from build123d import *

# Parameters (mm, degrees)
SKETCH2_W                       = 125
SKETCH2_H                       = 35
SKETCH2_R                       = 10
BOSS_EXTRUDE1_DEPTH             = 5
BOSS_EXTRUDE3_REACH             = 19.5
BOSS_EXTRUDE3_DIRECTION_2_REACH = 19.5
CUT_EXTRUDE2_DEPTH              = 12.5
CUT_EXTRUDE2_DEPTH_BACK         = 12.5
SKETCH8_R                       = 12.75
SKETCH8_R_2                     = 10.25
BOSS_EXTRUDE4_DEPTH             = 30.2
FILLET1_R                       = 5
SKETCH9_R                       = 3.5
CUT_EXTRUDE3_DEPTH              = 36.0000001
SKETCH13_R                      = 2
CUT_EXTRUDE5_DEPTH              = 2.5
CUT_EXTRUDE6_DEPTH              = 6
BOSS_EXTRUDE7_DEPTH             = 72
SKETCH17_R                      = 7.5
BOSS_EXTRUDE8_DEPTH             = 4
SKETCH18_R                      = 10.25
BOSS_EXTRUDE9_DEPTH             = 9.5


with BuildPart() as part:
    # Sketch2 → Boss-Extrude1 (new body)
    with BuildSketch(Plane(origin=(0, 0, 0), x_dir=(1, 0, 0), z_dir=(0, 1, 0))):
        Rectangle(SKETCH2_W, SKETCH2_H)
        with Locations((-25, 0)):
            Circle(SKETCH2_R, mode=Mode.SUBTRACT)
    extrude(amount=BOSS_EXTRUDE1_DEPTH)

    # Boss-Extrude3: up to this face of the body (flat: up to its plane)
    boss_extrude3_end = Plane(part.part.faces().sort_by_distance((0, 2.5, -17.5))[0])
    # Sketch6 → Boss-Extrude3 (add, up to the picked face)
    with BuildSketch(Plane.XY, mode=Mode.PRIVATE) as boss_extrude3_sk1:
        with BuildLine():
            Line((-62.5, 5), (-4.580943715, 34.11344911))
            ThreePointArc((-4.580943715, 34.11344911), (0, 35.2), (4.580943715, 34.11344911))
            Line((4.580943715, 34.11344911), (62.5, 5))
            Line((62.5, 5), (-62.5, 5))
        make_face()
    boss_extrude3_tool1 = split(extrude(boss_extrude3_sk1.sketch, amount=-BOSS_EXTRUDE3_REACH, mode=Mode.PRIVATE), bisect_by=boss_extrude3_end, keep=Keep.BOTH, mode=Mode.PRIVATE)
    add(boss_extrude3_tool1.solids().sort_by_distance((0, 15.43289, 0))[0])

    # Boss-Extrude3 direction 2: up to this face of the body (flat: up to its plane)
    boss_extrude3_direction_2_end = Plane(part.part.faces().sort_by_distance((0, 2.5, 17.5))[0])
    # Sketch6 → Boss-Extrude3 direction 2 (add, up to the picked face)
    with BuildSketch(Plane.XY, mode=Mode.PRIVATE) as boss_extrude3_direction_2_sk1:
        with BuildLine():
            Line((-62.5, 5), (-4.580943715, 34.11344911))
            ThreePointArc((-4.580943715, 34.11344911), (0, 35.2), (4.580943715, 34.11344911))
            Line((4.580943715, 34.11344911), (62.5, 5))
            Line((62.5, 5), (-62.5, 5))
        make_face()
    boss_extrude3_direction_2_tool1 = split(extrude(boss_extrude3_direction_2_sk1.sketch, amount=BOSS_EXTRUDE3_DIRECTION_2_REACH, mode=Mode.PRIVATE), bisect_by=boss_extrude3_direction_2_end, keep=Keep.BOTH, mode=Mode.PRIVATE)
    add(boss_extrude3_direction_2_tool1.solids().sort_by_distance((0, 15.43289, 0))[0])

    # Sketch7 → Cut-Extrude2 (cut, two sides)
    with BuildSketch(Plane.XY) as cut_extrude2_sk:
        with BuildLine():
            Line((4.580943715, 34.11344911), (62.5, 5))
            Line((62.5, 5), (-62.5, 5))
            Line((-62.5, 5), (-4.580943715, 34.11344911))
            ThreePointArc((-4.580943715, 34.11344911), (0, 35.2), (4.580943715, 34.11344911))
        make_face()
    extrude(amount=CUT_EXTRUDE2_DEPTH, mode=Mode.SUBTRACT)
    extrude(cut_extrude2_sk.sketch, amount=-CUT_EXTRUDE2_DEPTH_BACK, mode=Mode.SUBTRACT)

    # Sketch8 → Boss-Extrude4 (add)
    with BuildSketch(Plane(origin=(0, 5, 0), x_dir=(1, 0, 0), z_dir=(0, 1, 0))):
        Circle(SKETCH8_R)
        Circle(SKETCH8_R_2, mode=Mode.SUBTRACT)
    extrude(amount=BOSS_EXTRUDE4_DEPTH)

    # Fillet1
    fillet1_edges = [part.edges().sort_by_distance(p)[0] for p in [
        (0, 0, -17.5),
        (0, 0, 17.5),
    ]]
    fillet(fillet1_edges, radius=FILLET1_R)

    # Sketch9 → Cut-Extrude3 (cut, through all)
    with BuildSketch(Plane.XY.offset(17.5)):
        with Locations((0, 25)):
            Circle(SKETCH9_R)
    extrude(amount=-CUT_EXTRUDE3_DEPTH, mode=Mode.SUBTRACT)

    # Sketch13 → Cut-Extrude5 (cut)
    with BuildSketch(Plane(origin=(0, 5, 0), x_dir=(1, 0, 0), z_dir=(0, 1, 0))):
        with BuildLine():
            Line((23.5, 7.5), (53.5, 7.5))
            ThreePointArc((53.5, 7.5), (61, 0), (53.5, -7.5))
            Line((53.5, -7.5), (23.5, -7.5))
            ThreePointArc((23.5, -7.5), (16, 0), (23.5, 7.5))
        make_face()
        with Locations((31.5, 0)):
            Circle(SKETCH13_R, mode=Mode.SUBTRACT)
        with Locations((24.5, 0)):
            Circle(SKETCH13_R, mode=Mode.SUBTRACT)
        with Locations((38.5, 0)):
            Circle(SKETCH13_R, mode=Mode.SUBTRACT)
        with Locations((45.5, 0)):
            Circle(SKETCH13_R, mode=Mode.SUBTRACT)
        with Locations((52.5, 0)):
            Circle(SKETCH13_R, mode=Mode.SUBTRACT)
    extrude(amount=-CUT_EXTRUDE5_DEPTH, mode=Mode.SUBTRACT)

    # Sketch15 → Cut-Extrude6 (cut, through all)
    with BuildSketch(Plane(origin=(0, 5, 0), x_dir=(1, 0, 0), z_dir=(0, 1, 0))):
        with BuildLine():
            Line((23.5, 4), (53.5, 4))
            Line((53.5, 4), (62.5, 4))
            Line((62.5, 4), (62.5, -4))
            Line((62.5, -4), (53.5, -4))
            Line((53.5, -4), (23.5, -4))
            ThreePointArc((23.5, -4), (19.5, 0), (23.5, 4))
        make_face()
    extrude(amount=-CUT_EXTRUDE6_DEPTH, mode=Mode.SUBTRACT)

    # Sketch16 → Boss-Extrude7 (add)
    with BuildSketch(Plane(origin=(0, 5, 0), x_dir=(1, 0, 0), z_dir=(0, 1, 0))):
        with BuildLine():
            Line((16, -4), (16, -6.614378278))
            ThreePointArc((16, -6.614378278), (19.385621722, -9.114378278), (23.5, -10))
            Line((23.5, -10), (53.5, -10))
            Line((53.5, -10), (53.5, -7.5))
            Line((53.5, -7.5), (23.5, -7.5))
            ThreePointArc((23.5, -7.5), (19.877155813, -6.566962768), (17.15571123, -4))
            Line((17.15571123, -4), (16, -4))
        make_face()
        with BuildLine():
            Line((53.5, 10), (23.5, 10))
            ThreePointArc((23.5, 10), (19.385621722, 9.114378278), (16, 6.614378278))
            Line((16, 6.614378278), (16, 4))
            Line((16, 4), (17.15571123, 4))
            ThreePointArc((17.15571123, 4), (19.877155813, 6.566962768), (23.5, 7.5))
            Line((23.5, 7.5), (53.5, 7.5))
            Line((53.5, 7.5), (53.5, 10))
        make_face()
    extrude(amount=BOSS_EXTRUDE7_DEPTH)

    # Sketch17 → Boss-Extrude8 (add)
    with BuildSketch(Plane(origin=(0, 77, 0), x_dir=(1, 0, 0), z_dir=(0, 1, 0))):
        with BuildLine():
            Line((23.5, -10), (53.5, -10))
            ThreePointArc((53.5, -10), (63.5, 0), (53.5, 10))
            Line((53.5, 10), (23.5, 10))
            ThreePointArc((23.5, 10), (19.385621722, 9.114378278), (16, 6.614378278))
            Line((16, 6.614378278), (16, 4))
            Line((16, 4), (16, -4))
            Line((16, -4), (16, -6.614378278))
            ThreePointArc((16, -6.614378278), (19.385621722, -9.114378278), (23.5, -10))
        make_face()
        with Locations((38.5, 0)):
            Circle(SKETCH17_R, mode=Mode.SUBTRACT)
    extrude(amount=BOSS_EXTRUDE8_DEPTH)

    # Sketch18 → Boss-Extrude9 (add)
    with BuildSketch(Plane(origin=(0, 5, 0), x_dir=(1, 0, 0), z_dir=(0, 1, 0))):
        Circle(SKETCH18_R)
    extrude(amount=BOSS_EXTRUDE9_DEPTH)


solid = part.part
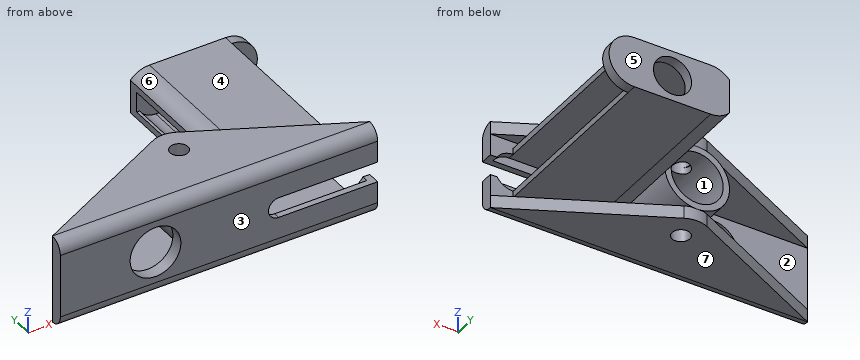
Could you check a few things on this model? Use its own coordinates, in mm. Face numbers are marked on the shaded views. A direction names the side the tool comes from. Coordinates: 2 decimals unless noted, no trailing zeros. Loops run counter-clockwise (first coordinate to the right, second up) from the corner with the lowest first, then second, coordinate; pieces in that order, holes last.
1. Imagine slicing it at A-A (y = 57.5). Please give me the cut outline in (x, z).
2. I need wall thicknesses on L1, parallel to Z at x = 38, y = 78; L2, parallel to Y at x = 50, z = 4.5; L3, parallel to Z at x = 20.5, y = 7. Which ranges of each line are inside material? Lowest first, please.
3. We'd pull the mould along X, two halves only. Please class the marked faces 6 and 7: released by +X, released by -X, zero draft, split by the parting line, or undercut.
4. For P1, Ø10, axis at y = 67.5, z = 12, coming from the -X side; P2, Ø12, axis at x = 49, y = 59.5, coming from the +Z side; P3, Ø1.5, axis at x = 52.5, y = 2.5, coming from the -Z side, each with a flat end and sliding along its axis, tell me the tip position at first contact or that it passes through.
5. Imagine slicing it at D-D (x = -49). Please give me the cut outline in (y, z), and give its area (3 significant figures).
6. For the marked faces 1, 2, 3, 4 and 5, which set-ups out of +Z, -Z, +X, -X, +Y, -Y let a thin tool reach every point of the face, with its end or its side?
7. Imagine slicing it at B-B (x = -28). Please give me the cut outline in (y, z).
8. Imagine slicing it at C-C (z = 0). Please give me the cut outline in (x, y), and give its area (3 significant figures).
Computed values:
1. outline: (16, -6.61) arc R10 ccw to (23.5, -10) - (53.5, -10) - (53.5, -7.5) - (23.5, -7.5) arc R7.5 cw to (17.16, -4) - (16, -4) - close; (16, 4) - (17.16, 4) arc R7.5 cw to (23.5, 7.5) - (53.5, 7.5) - (53.5, 10) - (23.5, 10) arc R10 ccw to (16, 6.61) - close
2. L1: z = -10 to -7.48, 7.48 to 10
2. L2: y = 0 to 2.5, 77 to 81
2. L3: z = -17.5 to -12.5, -9.54 to -6.87, 6.87 to 9.54, 12.5 to 17.5
3. face 6: undercut
3. face 7: zero draft
4. P1: stops at x = 16.36
4. P2: stops at z = 10
4. P3: stops at z = -17.18
5. outline: (0, -12.5) arc R5 ccw to (5, -17.5) - (11.79, -17.5) - (11.79, -12.5) - (5, -12.5) - (5, 12.5) - (11.79, 12.5) - (11.79, 17.5) - (5, 17.5) arc R5 ccw to (0, 12.5) - close
5. area: 232 mm2
6. face 1: +Y
6. face 2: -X, +Y
6. face 3: +Z, -Z, +X, -X, -Y
6. face 4: +X, +Y
6. face 5: +Z, -Z, +X, -X, +Y
7. outline: (0, -12.5) arc R5 ccw to (5, -17.5) - (22.34, -17.5) - (22.34, -12.5) - (5, -12.5) - (5, -9.54) - (0, -9.54) - close; (0, 9.54) - (5, 9.54) - (5, 12.5) - (22.34, 12.5) - (22.34, 17.5) - (5, 17.5) arc R5 ccw to (0, 12.5) - close
8. outline: (-62.5, 0) - (-35, 0) - (-35, 5) - (-62.5, 5) - close; (-15, 0) - (19.5, 0) - (19.5, 2.5) - (16, 2.5) - (16, 5) - (12.75, 5) - (12.75, 35.2) - (10.25, 35.2) - (10.25, 14.5) - (-10.25, 14.5) - (-10.25, 35.2) - (-12.75, 35.2) - (-12.75, 5) - (-15, 5) - close; (16, 77) - (31, 77) - (31, 81) - (16, 81) - close; (46, 77) - (63.5, 77) - (63.5, 81) - (46, 81) - close
8. area: 777 mm2
